```python
from build123d import *

# Parameters (mm, degrees)
EXTRUDE_1_DEPTH             = 5.8
EXTRUDE_1_DEPTH_BACK        = 5.8
SKETCH_1_W                  = 17.3
SKETCH_1_H                  = 10.8
EXTRUDE_2_DEPTH             = 7.5
EXTRUDE_2_DEPTH_BACK        = 7.5
CHAMFER_1_SIZE              = 1.5
EXTRUDE_3_DEPTH             = 5
EXTRUDE_3_DEPTH_BACK        = 5
EXTRUDE_4_REACH             = 23.183
SKETCH_4_W                  = 18.6
SKETCH_4_H                  = 2
EXTRUDE_4_DIRECTION_2_REACH = 23.183
EXTRUDE_5_DEPTH             = 2.7
EXTRUDE_5_DEPTH_BACK        = 2.7
SKETCH_5_W                  = 0.5
SKETCH_5_H                  = 7.4
SKETCH_6_R                  = 0.75
SKETCH_6_R_2                = 1
CUT_EXTRUDE_1_DEPTH         = 26.738881095


with BuildPart() as part:
    # Sketch 1 → Extrude 1 (new, two sides: drawn at the far end of the back side and taken through both)
    with BuildSketch(Plane.XY.offset(-EXTRUDE_1_DEPTH_BACK)):
        with Locations((0, 5.4)):
            Rectangle(SKETCH_1_W, SKETCH_1_H)
    extrude(amount=EXTRUDE_1_DEPTH + EXTRUDE_1_DEPTH_BACK)

    # Sketch 2 → Extrude 2 (add, two sides: drawn at the far end of the back side and taken through both)
    with BuildSketch(Plane.XY.offset(-EXTRUDE_2_DEPTH_BACK)):
        Polygon((-8.5, 12.8), (-10.5, 11.3), (-10.5, 10.8), (10.5, 10.8), (10.5, 11.3), (8.5, 12.8), align=None)
    extrude(amount=EXTRUDE_2_DEPTH + EXTRUDE_2_DEPTH_BACK)

    # Chamfer 1
    chamfer_1_edges = [part.edges().sort_by_distance(p)[0] for p in [
        (0, 12.8, -7.5),
        (0, 12.8, 7.5),
    ]]
    chamfer(chamfer_1_edges, length=CHAMFER_1_SIZE)

    # Sketch 3 → Extrude 3 (add, two sides: drawn at the far end of the back side and taken through both)
    with BuildSketch(Plane.XY.offset(-EXTRUDE_3_DEPTH_BACK)):
        with BuildLine():
            ThreePointArc((-4.5, 16.8), (-6.57373706, 15.230302795), (-7.5, 12.8))
            Line((-7.5, 12.8), (7.5, 12.8))
            ThreePointArc((7.5, 12.8), (1.17544468, 13.826334039), (-4.5, 16.8))
        make_face()
    extrude(amount=EXTRUDE_3_DEPTH + EXTRUDE_3_DEPTH_BACK)

    # Extrude 4: up to this face of the body (flat: up to its plane)
    extrude_4_end = Plane(part.part.faces().sort_by_distance((0, 5.4, 5.8))[0])
    # Sketch 4 → Extrude 4 (add, up to the picked face)
    with BuildSketch(Plane.XY, mode=Mode.PRIVATE) as extrude_4_sk1:
        with Locations((0, 1)):
            Rectangle(SKETCH_4_W, SKETCH_4_H)
    extrude_4_tool1 = split(extrude(extrude_4_sk1.sketch, amount=EXTRUDE_4_REACH, mode=Mode.PRIVATE), bisect_by=extrude_4_end, keep=Keep.BOTH, mode=Mode.PRIVATE)
    add(extrude_4_tool1.solids().sort_by(Axis((0, 1, 0), (0, 0, 1)))[0])

    # Extrude 4 direction 2: up to this face of the body (flat: up to its plane)
    extrude_4_direction_2_end = Plane(part.part.faces().sort_by_distance((0, 5.4, -5.8))[0])
    # Sketch 4 → Extrude 4 direction 2 (add, up to the picked face)
    with BuildSketch(Plane.XY, mode=Mode.PRIVATE) as extrude_4_direction_2_sk1:
        with Locations((0, 1)):
            Rectangle(SKETCH_4_W, SKETCH_4_H)
    extrude_4_direction_2_tool1 = split(extrude(extrude_4_direction_2_sk1.sketch, amount=-EXTRUDE_4_DIRECTION_2_REACH, mode=Mode.PRIVATE), bisect_by=extrude_4_direction_2_end, keep=Keep.BOTH, mode=Mode.PRIVATE)
    add(extrude_4_direction_2_tool1.solids().sort_by(Axis((0, 1, 0), (0, 0, -1)))[0])

    # Sketch 5 → Extrude 5 (add, two sides: drawn at the far end of the back side and taken through both)
    with BuildSketch(Plane.XY.offset(-EXTRUDE_5_DEPTH_BACK)):
        Polygon((-9.3, 2), (-10.7, 7.5), (-10.15, 10.3), (-9.130890495, 10.3), (-9.168751179, 10.107254696), (-9.675324513, 7.528335908), (-8.65, 3.500275321), (-8.65, 2), align=None)
        Polygon((8.65, 2), (8.65, 3.500275321), (9.675324513, 7.528335908), (9.168751179, 10.107254696), (9.130890495, 10.3), (10.15, 10.3), (10.7, 7.5), (9.3, 2), align=None)
        with Locations((0, -3.7)):
            Rectangle(SKETCH_5_W, SKETCH_5_H)
        with Locations((-7.05, -3.7)):
            Rectangle(SKETCH_5_W, SKETCH_5_H)
        with Locations((7.05, -3.7)):
            Rectangle(SKETCH_5_W, SKETCH_5_H)
    extrude(amount=EXTRUDE_5_DEPTH + EXTRUDE_5_DEPTH_BACK)

    # Sketch 6 → Cut-Extrude 1 (cut, through all)
    with BuildSketch(Plane.ZY.offset(7.3)):
        with Locations(Location((0, -0.9, 0), (0, 0, 270))):
            Circle(SKETCH_6_R)
        Polygon((-1.2, -7.4), (-2.7, -5.9), (-2.7, -7.4), align=None)
        Polygon((2.7, -5.9), (1.2, -7.4), (2.7, -7.4), align=None)
        with Locations(Location((0, -4.9, 0), (0, 0, 270))):
            Circle(SKETCH_6_R_2)
    extrude(amount=-CUT_EXTRUDE_1_DEPTH, mode=Mode.SUBTRACT)


solid = part.part
```
The model under review builds one solid part; all positions refer to its coordinate system, in mm. A direction names the side the tool comes from. Round coordinates to 2 decimals unless told otherwise and drop trailing zeros. Order: outer loops, then holes, each group sorted by start corner. A loop starts at its lowest first (then second) coordinate and runs counter-clockwise, first axis right, second up.
(1) Wall thickness on L1, parallel to X at y = 10.25, z = -1; L2, parallel to Z at x = 7.1, y = -4.9; L3, parallel to Y at x = -8.75, z = -2.75: over which ranges is each line inside the solid? List them lowest first.
Working result:
L1: x = -10.16 to -9.14, -8.65 to 8.65, 9.14 to 10.16
L2: z = -2.7 to -1, 1 to 2.7
L3: y = 0 to 2, 10.8 to 12.61
(2) Tool access review of faces 4 (the face through (0, 12.8, -5.4)), 5 (the face through (-3, 14, 5)), 6 (the face through (0, 5, 5.8)), 7 (the face through (-10, 10.3, 0)), 8 (the face through (6.8, -3.75, -0.04)): name each direction out of +Z, -Z, +X, -X, +Y, -Y from which nothing blocks a thin tool from reaching the whole face with its end or side.
Working result:
face 4: +Y
face 5: +Z, +X, -X, +Y
face 6: +Z, +X, -X, -Y
face 7: +Z, -Z, -X
face 8: +Z, -Z, -Y
(3) Mouldability with a two-part tool opening along X and no side actions: class faces 1 (the face through (-9.486, 12.061, -0.105)), 2 (the face through (-0.25, -3.75, -0.04)), 3 (the face through (7, -6.6, 2)) as released by +X, released by -X, zero draft, split by the parting line, or undercut.
Working result:
face 1: released by -X
face 2: undercut
face 3: zero draft
(4) For P1, Ø4, axis at x = -7.5, z = 5.5, coming from the -Y side; P2, Ø4, axis at x = 2, z = 2, coming from the +Y side; P3, Ø7, axis at y = 7, z = 1.5, coming from the -X side; P4, Ø1, axis at x = 7.5, y = -2, coming from the -Z side, all flat-tipped, find the tip position at first contact; note any pin that passes through.
Working result:
P1: stops at y = 0
P2: stops at y = 14.26
P3: stops at x = -10.7
P4: stops at z = -2.7
(5) Take a section at C-C, the plane z = 0. Count the separate pieces of the cut face and the enclosed holes in it, plus the area to 3 significant figures.
Working result:
separate pieces: 7
enclosed holes: 0
area: 275 mm2
(6) Take a section at A-A, the plane y = -0.9. State the section outline as (x, z) points.
Working result:
outline: (-7.3, -2.7) - (-6.8, -2.7) - (-6.8, -0.75) - (-7.3, -0.75) - close; (-7.3, 0.75) - (-6.8, 0.75) - (-6.8, 2.7) - (-7.3, 2.7) - close; (-0.25, -2.7) - (0.25, -2.7) - (0.25, -0.75) - (-0.25, -0.75) - close; (-0.25, 0.75) - (0.25, 0.75) - (0.25, 2.7) - (-0.25, 2.7) - close; (6.8, -2.7) - (7.3, -2.7) - (7.3, -0.75) - (6.8, -0.75) - close; (6.8, 0.75) - (7.3, 0.75) - (7.3, 2.7) - (6.8, 2.7) - close
(7) Take a section at D-D, the plane y = -4.9. State the section outline as (x, z) points, plus the area to 3 significant figures.
Working result:
outline: (-7.3, -2.7) - (-6.8, -2.7) - (-6.8, -1) - (-7.3, -1) - close; (-7.3, 1) - (-6.8, 1) - (-6.8, 2.7) - (-7.3, 2.7) - close; (-0.25, -2.7) - (0.25, -2.7) - (0.25, -1) - (-0.25, -1) - close; (-0.25, 1) - (0.25, 1) - (0.25, 2.7) - (-0.25, 2.7) - close; (6.8, -2.7) - (7.3, -2.7) - (7.3, -1) - (6.8, -1) - close; (6.8, 1) - (7.3, 1) - (7.3, 2.7) - (6.8, 2.7) - close
area: 5.10 mm2
(8) Take a section at B-B, the plane z = -5.5. State the section outline as (x, y) points.
Working result:
outline: (-10.5, 10.8) - (-8.65, 10.8) - (-8.65, 2) - (-9.3, 2) - (-9.3, 0) - (9.3, 0) - (9.3, 2) - (8.65, 2) - (8.65, 10.8) - (10.5, 10.8) - (10.5, 11.3) - (8.5, 12.8) - (-8.5, 12.8) - (-10.5, 11.3) - close
